Verification items for the finished model (mm, model axes). Give positions to 0.01 mm unless a question says otherwise; leave off trailing zeros. Order: outer loops, then holes, each group sorted by start corner. A loop starts at its lowest first (then second) coordinate and runs counter-clockwise, first axis right, second up. Notation, with made-up numbers: (47.25, 2.5) - (93.25, 2.5) arc R25 ccw to (93.25, 37.5) - close; hole circle Ø5 at (38, -29.75). An arc over 180 degrees is marked (long way). Answer as a JSON object with one key per item and string values. Group by question number.
(1) Section check A-A (x = 0). Record the boundary of the cut face in (y, z), then the cut area to 3 significant figures.
(2) Section check D-D (y = -10.05). Record the boundary of the cut face in (x, z), then the cut area to 3 significant figures.
(3) Section check B-B (x = 31). Record the boundary of the cut face in (y, z), then the cut area to 3 significant figures.
(4) Section check C-C (z = 1). Count the separate pieces of the cut face and the enclosed holes in it, then the cut area to 3 significant figures.
(5) Depth check by flat-ended pin: pin 1 Ø0.6 at (y, z) = (-9.5, 1) entering from +X; pin 2 Ø1 at (y, z) = (-9.5, 0.5) entering from +X; pin 3 Ø1 at (y, z) = (10.5, 1.5) entering from -X. Enter the tip coordinate at first touch or a pass-through.
(6) Thickness scan on line 1 (Y direction, x = 0, z = 1.7); line 2 (Y direction, x = -17, z = 0.75); line 3 (Y direction, x = -15, z = 1.05). Record the ranges inside material, lowest first.
```python
from build123d import *

# Parameters (mm, degrees)
SKETCH_1_R      = 5.05
SKETCH_1_R_2    = 2.05
SKETCH_1_R_3    = 1.15
SKETCH_1_W      = 8.1
SKETCH_1_H      = 2.1
EXTRUDE_1_DEPTH = 2


with BuildPart() as part:
    # 草图1 → 凸台-拉伸1 (new body)
    with BuildSketch(Plane.XY):
        with BuildLine():
            ThreePointArc((-7.35497191, -38.809204942), (0, 39.5), (7.35497191, -38.809204942))
            ThreePointArc((7.35497191, -38.809204942), (0, -27.662081143), (-7.35497191, -38.809204942))
        make_face()
        Circle(SKETCH_1_R, mode=Mode.SUBTRACT)
        with Locations((-17.67766953, -17.67766953)):
            Circle(SKETCH_1_R_2, mode=Mode.SUBTRACT)
        with Locations((-17.67766953, 17.67766953)):
            Circle(SKETCH_1_R_2, mode=Mode.SUBTRACT)
        with Locations((17.67766953, 17.67766953)):
            Circle(SKETCH_1_R_2, mode=Mode.SUBTRACT)
        with Locations((17.67766953, -17.67766953)):
            Circle(SKETCH_1_R_2, mode=Mode.SUBTRACT)
        with Locations((31, 10.05)):
            Circle(SKETCH_1_R_2, mode=Mode.SUBTRACT)
        with Locations(Location((31, -10.05, 0), (0, 0, 180))):
            Circle(SKETCH_1_R_2, mode=Mode.SUBTRACT)
        with Locations((-31, -10.05)):
            Circle(SKETCH_1_R_2, mode=Mode.SUBTRACT)
        with Locations(Location((-31, 10.05, 0), (0, 0, 180))):
            Circle(SKETCH_1_R_2, mode=Mode.SUBTRACT)
        with Locations((-14.05, 0)):
            Circle(SKETCH_1_R_3, mode=Mode.SUBTRACT)
        with Locations((14.05, 0)):
            Circle(SKETCH_1_R_3, mode=Mode.SUBTRACT)
        with Locations((16, -10.05)):
            Rectangle(SKETCH_1_W, SKETCH_1_H, mode=Mode.SUBTRACT)
        with Locations((16, 10.05)):
            Rectangle(SKETCH_1_W, SKETCH_1_H, mode=Mode.SUBTRACT)
        with Locations((-16, 10.05)):
            Rectangle(SKETCH_1_W, SKETCH_1_H, mode=Mode.SUBTRACT)
        with Locations((-16, -10.05)):
            Rectangle(SKETCH_1_W, SKETCH_1_H, mode=Mode.SUBTRACT)
    extrude(amount=EXTRUDE_1_DEPTH)


solid = part.part
```
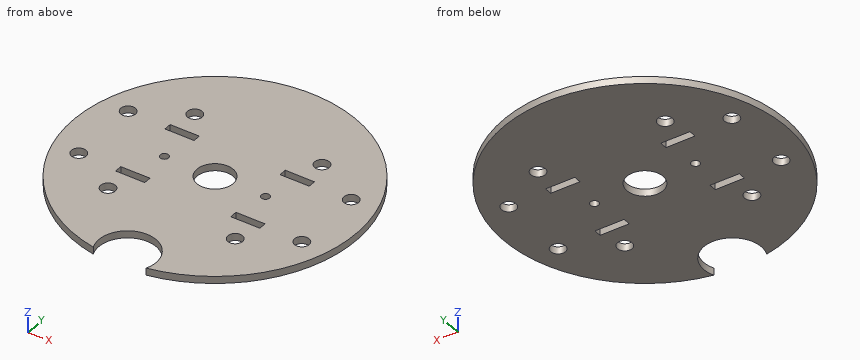
Solutions:
{
 "1": {"outline": "(-27.66, 0) - (-5.05, 0) - (-5.05, 2) - (-27.66, 2) - close; (5.05, 0) - (39.5, 0) - (39.5, 2) - (5.05, 2) - close", "area": "114 mm2"},
 "2": {"outline": "(-38.2, 0) - (-33.05, 0) - (-33.05, 2) - (-38.2, 2) - close; (-28.95, 0) - (-20.05, 0) - (-20.05, 2) - (-28.95, 2) - close; (-11.95, 0) - (11.95, 0) - (11.95, 2) - (-11.95, 2) - close; (20.05, 0) - (28.95, 0) - (28.95, 2) - (20.05, 2) - close; (33.05, 0) - (38.2, 0) - (38.2, 2) - (33.05, 2) - close", "area": "104 mm2"},
 "3": {"outline": "(-24.48, 0) - (-12.1, 0) - (-12.1, 2) - (-24.48, 2) - close; (-8, 0) - (8, 0) - (8, 2) - (-8, 2) - close; (12.1, 0) - (24.48, 0) - (24.48, 2) - (12.1, 2) - close", "area": "81.5 mm2"},
 "4": {"separate pieces": "1", "enclosed holes": "15", "area": "4,480 mm2"},
 "5": {"pin 1": "stops at x = 38.41", "pin 2": "stops at x = 38.46", "pin 3": "stops at x = -38.21"},
 "6": {"line 1": "y = -27.66 to -5.05, 5.05 to 39.5", "line 2": "y = -35.65 to -19.61, -15.74 to -11.1, -9 to 9, 11.1 to 15.74, 19.61 to 35.65", "line 3": "y = -36.54 to -11.1, -9 to -0.65, 0.65 to 9, 11.1 to 36.54"}
}
